Answer from the drawing. Dimensions are ordinates in mm from the lowest x, y and z of the part. A direction names the side the tool comes from. Give positions to 0.01 mm unless a question says otherwise; leave off trailing zeros. Order: outer loops, then holes, each group sorted by start corner. A loop starts at its lowest first (then second) coordinate and runs counter-clockwise, first axis right, second up. Notation, with made-up numbers: M 24,-15.75 L 69,-15.75 A17 cw 69,13.25 Z; hole C 3.25,-22 d1. An arc over 180 degrees is marked long. One line per item, written item: value.
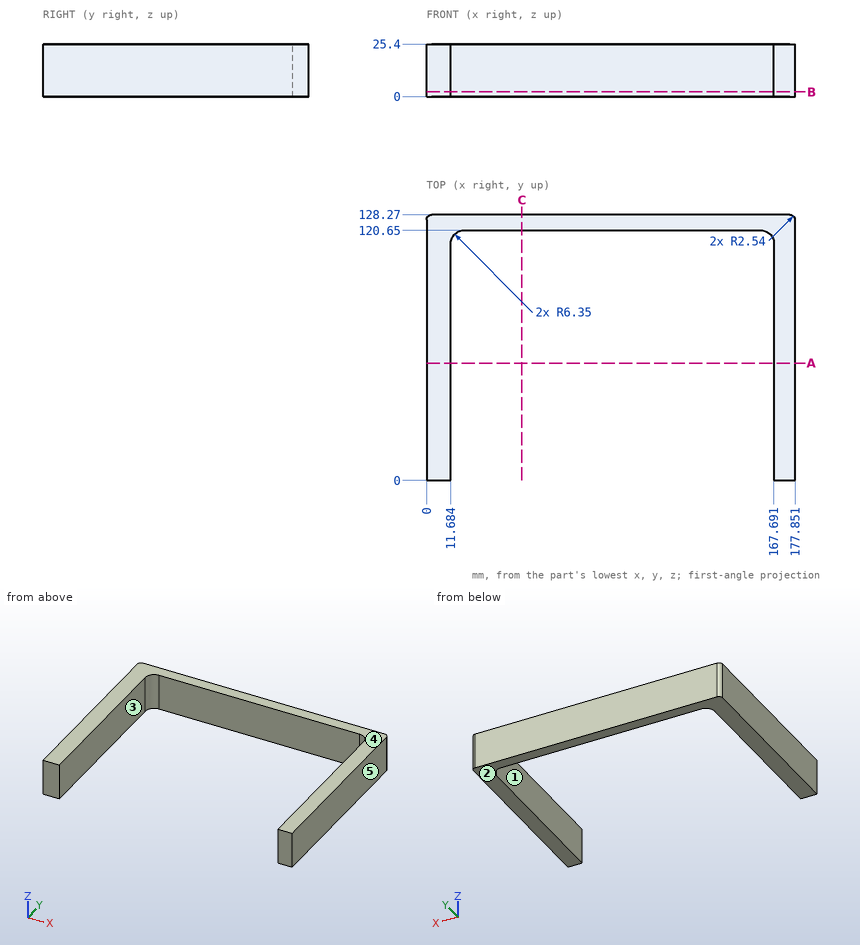
(1) Section A-A, the plane y = 56.5 is taken. Give the vertices of the cut face in (x, z), then the cut area to 3 significant figures.
Findings:
outline: M 0,0 L 11.68,0 L 11.68,25.4 L 0,25.4 Z; M 167.69,0 L 177.85,0 L 177.85,25.4 L 167.69,25.4 Z
area: 555 mm^2
(2) Which of the six approach directions +Z, -Z, +X, -X, +Y, -Y give full straight-line access (tool end or side, diameter ignored) to the marked faces 1 and 2?
Findings:
face 1: +Z, -Z, -Y
face 2: -Z, +X, -X, +Y, -Y
(3) Section B-B, the plane z = 2.25 is taken. Give the vertices of the cut face in (x, y).
Findings:
outline: M 0,0 L 11.68,0 L 11.68,114.3 A6.35 cw 18.03,120.65 L 161.34,120.65 A6.35 cw 167.69,114.3 L 167.69,0 L 177.85,0 L 177.85,125.73 A2.54 ccw 175.31,128.27 L 2.54,128.27 A2.54 ccw 0,125.73 Z
(4) Determine the mould class of the marked faces 3, 4 and 5 for opening direction X: pulls with the +X half, pulls with the -X half, needs draft (parallel to the pull), parting line crosses it, or undercut.
Findings:
face 3: undercut
face 4: needs draft
face 5: pulls with the +X half
(5) Given P1, Ø12.5, axis at x = 102.5, z = 11.5, coming from the -Y side; P2, Ø10, axis at y = 79, z = 9.5, coming from the -X side, each flat-ended and moving along its own axis, determine where each tip first touches the part or whether it passes through.
Findings:
P1: stops at y = 120.65
P2: stops at x = 0
(6) Find the intervals of material crossed by probe 1 along X at (y, z) = (44, 13.25); probe 2 along Y at (x, z) = (152, 16); probe 3 along Y at (x, z) = (164, 15.25), in increasing order. Write a range as from..to.
Findings:
probe 1: x = 0..11.68, 167.69..177.85
probe 2: y = 120.65..128.27
probe 3: y = 120.07..128.27
(7) Section C-C, the plane x = 46 is taken. Give the vertices of the cut face in (y, z), then the cut area to 3 significant figures.
Findings:
outline: M 120.65,0 L 128.27,0 L 128.27,25.4 L 120.65,25.4 Z
area: 194 mm^2
